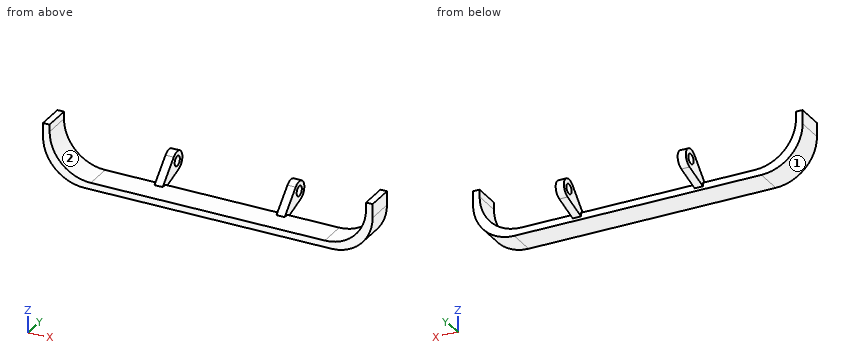
```python
from build123d import *

# Parameters (mm, degrees)
BOSS_EXTRUDE1_DEPTH  = 10
SKETCH2_R            = 3.55
SKETCH2_R_2          = 1.75
BOSS_EXTRUDE2_DEPTH  = 3
BOSS_EXTRUDE3_START  = -44.4
SKETCH2_3_R          = 3.55
SKETCH2_3_R_2        = 1.75
BOSS_EXTRUDE3_DEPTH  = 3
M3_CLEARANCE_HOLE1_D = 3.6


with BuildPart() as part:
    # Sketch1 → Boss-Extrude1 (new body)
    with BuildSketch(Plane(origin=(0, 0, 0), x_dir=(1, 0, 0), z_dir=(0, 1, 0))):
        with BuildLine():
            Line((0, 0), (0, 5))
            ThreePointArc((0, 5), (4.393398282, 15.606601718), (15, 20))
            Line((15, 20), (105, 20))
            ThreePointArc((105, 20), (115.606601718, 15.606601718), (120, 5))
            Line((120, 5), (120, 0))
            Line((120, 0), (117.6, 0))
            Line((117.6, 0), (117.6, 2.6))
            ThreePointArc((117.6, 2.6), (113.206601718, 13.206601718), (102.6, 17.6))
            Line((102.6, 17.6), (17.4, 17.6))
            ThreePointArc((17.4, 17.6), (6.793398282, 13.206601718), (2.4, 2.6))
            Line((2.4, 2.6), (2.4, 0))
            Line((2.4, 0), (0, 0))
        make_face()
    extrude(amount=BOSS_EXTRUDE1_DEPTH)

    # Sketch2 → Boss-Extrude2 (add)
    # profile 1 of 3: a face of its own
    with BuildSketch(Plane(origin=(80.7, 0, 0), x_dir=(0, 0, -1), z_dir=(1, 0, 0))):
        with BuildLine():
            Line((17.6, 10), (18.9, 10))
            Line((18.9, 10), (16.218619991, 19.284947678))
            ThreePointArc((16.218619991, 19.284947678), (16.32297688, 18.797379809), (16.357992766, 18.3))
            ThreePointArc((16.357992766, 18.3), (14.134741273, 15.007244558), (10.249689442, 15.838784019))
            Line((10.249689442, 15.838784019), (17.6, 8.19852649))
            Line((17.6, 8.19852649), (17.6, 10))
        make_face()
    # profile 2 of 3: a face of its own
    with BuildSketch(Plane(origin=(80.7, 0, 0), x_dir=(0, 0, -1), z_dir=(1, 0, 0))):
        with Locations((12.807992766, 18.3)):
            Circle(SKETCH2_R)
        with Locations((12.807992766, 18.3)):
            Circle(SKETCH2_R_2, mode=Mode.SUBTRACT)
    # profile 3 of 3: a face of its own
    with BuildSketch(Plane(origin=(80.7, 0, 0), x_dir=(0, 0, -1), z_dir=(1, 0, 0))):
        with Locations((12.807992766, 18.3)):
            Circle(SKETCH2_R_2)
    extrude(amount=BOSS_EXTRUDE2_DEPTH)

    # Sketch2<3> → Boss-Extrude3 (add)
    with BuildSketch(Plane(origin=(80.7, 0, 0), x_dir=(0, 0, -1), z_dir=(1, 0, 0)).offset(BOSS_EXTRUDE3_START)):
        with BuildLine():
            Line((17.6, 10), (18.9, 10))
            Line((18.9, 10), (16.218619991, 19.284947678))
            ThreePointArc((16.218619991, 19.284947678), (16.32297688, 18.797379809), (16.357992766, 18.3))
            ThreePointArc((16.357992766, 18.3), (14.134741273, 15.007244558), (10.249689442, 15.838784019))
            Line((10.249689442, 15.838784019), (17.6, 8.19852649))
            Line((17.6, 8.19852649), (17.6, 10))
        make_face()
        with Locations((12.807992766, 18.3)):
            Circle(SKETCH2_3_R)
        with Locations((12.807992766, 18.3)):
            Circle(SKETCH2_3_R_2)
    extrude(amount=BOSS_EXTRUDE3_DEPTH)

    # M3 Clearance Hole1 (through all)
    with Locations(Plane(origin=(83.7, 0, 0), x_dir=(0, 0, -1), z_dir=(1, 0, 0))):
        with Locations((12.807992766, 18.3)):
            Hole(M3_CLEARANCE_HOLE1_D / 2)


solid = part.part
```
The model under review builds one solid part; all positions refer to its coordinate system, in mm. Face numbers are marked on the shaded views. A direction names the side the tool comes from. Round coordinates to 2 decimals unless told otherwise and drop trailing zeros. Order: outer loops, then holes, each group sorted by start corner. A loop starts at its lowest first (then second) coordinate and runs counter-clockwise, first axis right, second up. Notation, with made-up numbers: M 55.25,72 L 110.25,72 A19 cw 110.25,94 Z; hole C 34.25,-15.75 d10. An arc over 180 degrees is marked long. Use a Markdown table: item, result.
1) Wall thickness on line 1 along X through (y, z) = (15.25, -14.5); line 2 along X through (y, z) = (4.75, -1.75); line 3 along Z through (x, y) = (83, 1.75): over which ranges is each line inside the solid? List them lowest first. Write a range as [from, to].
Report:
| item | result |
|---|---|
| line 1 | [36.3, 39.3], [80.7, 83.7] |
| line 2 | [0, 2.4], [117.6, 120] |
| line 3 | [-20, -17.6] |
2) Consider section C-C (x = 46). Write out the cut boundary in (y, z), then the cut area to 3 significant figures.
Report:
| item | result |
|---|---|
| outline | M 0,-20 L 10,-20 L 10,-17.6 L 0,-17.6 Z |
| area | 24.0 mm^2 |
3) Tool access review of the marked faces 1 and 2: name each direction out of +Z, -Z, +X, -X, +Y, -Y from which nothing blocks a thin tool from reaching the whole face with its end or side.
Report:
| item | result |
|---|---|
| face 1 | -Z, -X, +Y, -Y |
| face 2 | +Z, +Y, -Y |
4) Insertion check: pin 1 (8 mm diameter, centred on x = 78.5, y = 2.5, fed in from +Z); pin 2 (8 mm diameter, centred on y = 19.5, z = -13, fed in from -X); pin 3 (3 mm diameter, centred on y = 18.3, z = -12.81, fed in from +X); pin 4 (6 mm diameter, centred on y = 19, z = -8, fed in from +X). Each pin has a flat end and moves straight along its axis. Give the tip position at first contact, or say it passes through.
Report:
| item | result |
|---|---|
| pin 1 | z = -17.6 |
| pin 2 | x = 36.3 |
| pin 3 | through |
| pin 4 | x = 83.7 |
5) Consider section A-A (y = 13.75). Write out the cut boundary in (x, z).
Report:
| item | result |
|---|---|
| outline | M 36.3,-17.82 L 39.3,-17.82 L 39.3,-12.26 L 36.3,-12.26 Z; M 80.7,-17.82 L 83.7,-17.82 L 83.7,-12.26 L 80.7,-12.26 Z |
6) Consider section B-B (y = 3.5). Write out the cut boundary in (x, z), then the cut area to 3 significant figures.
Report:
| item | result |
|---|---|
| outline | M 0,-5 A15 ccw 15,-20 L 105,-20 A15 ccw 120,-5 L 120,0 L 117.6,0 L 117.6,-2.6 A15 cw 102.6,-17.6 L 17.4,-17.6 A15 cw 2.4,-2.6 L 2.4,0 L 0,0 Z |
| area | 372 mm^2 |
